Here's how the part is built. I have some questions about the finished solid (model axes, mm). A direction names the side the tool comes from. Coordinates: 2 decimals unless noted, no trailing zeros. Write each loop counter-clockwise with the first axis right and the second up, starting at its lowest first coordinate (ties: lowest second). Pieces come first, ordered by that corner, then holes. Notation, with made-up numbers: (32.25, 24) -> (50.25, 24) arc R21 cw to (50.25, 60) -> close; hole circle Ø1 at (40, -6). An arc over 180 degrees is marked (long way). Put each result on its own line as item: value.
```python
from build123d import *

# Parameters (mm, degrees)
BOX007_W                  = 50
BOX007_H                  = 58
BOX007_DEPTH              = 50
BOX006_W                  = 50
BOX006_H                  = 50
BOX006_DEPTH              = 50
CUT002008_PLACEMENT_ANGLE = 180


with BuildPart() as cube002:
    # Box007 → Box007 (new body)
    with BuildSketch(Plane(origin=(5, -3, -5), x_dir=(1, 0, 0), z_dir=(0, 0, 1))):
        with Locations((25, 29)):
            Rectangle(BOX007_W, BOX007_H)
    extrude(amount=BOX007_DEPTH)


with BuildPart() as cut002008:
    # Box006 → Box006 (new body)
    with BuildSketch(Plane.XY):
        with Locations((25, 25)):
            Rectangle(BOX006_W, BOX006_H)
    extrude(amount=BOX006_DEPTH)

    # Cut002008: cut Cube002
    add(cube002.part, mode=Mode.SUBTRACT)


with BuildPart() as cut002008_1:
    # Cut002008 placement: moved
    add(cut002008.part.moved(Location((66, 35, 56))).rotate(Axis((66, 35, 56), (0, 1, 0)), CUT002008_PLACEMENT_ANGLE))


solid = cut002008_1.part
```
Item 1: Imagine slicing it at C-C on z = 37. Write out the boundary of the cut face in (x, y).
Output:
outline: (61, 35) -> (66, 35) -> (66, 85) -> (61, 85) -> close
Item 2: Imagine slicing it at A-A on y = 41. Write out the boundary of the cut face in (x, z), then the cut area to 3 significant figures.
Output:
outline: (16, 6) -> (66, 6) -> (66, 56) -> (61, 56) -> (61, 11) -> (16, 11) -> close
area: 475 mm²
Item 3: Imagine slicing it at B-B on x = 35. Write out the boundary of the cut face in (y, z).
Output:
outline: (35, 6) -> (85, 6) -> (85, 11) -> (35, 11) -> close
Item 4: Please list where these lines run through material, in increasing order: line 1 along X through (y, z) = (50.5, 32.5); line 2 along Z through (x, y) = (19, 48). Write a range as from..to.
Output:
line 1: x = 61..66
line 2: z = 6..11
Item 5: For P1, Ø4, axis at x = 57.5, z = 49, coming from the -Y side; P2, Ø1, axis at y = 61, z = 32.5, coming from the -X side; P3, Ø12, axis at x = 26.5, y = 42, coming from the +Z side, each with a flat end and sliding along its axis, tell me the tip position at first contact or that it passes through.
Output:
P1: passes through
P2: stops at x = 61
P3: stops at z = 11
Item 6: Which directions (+Z, -Z, +X, -X, +Y, -Y) give clear straight access to the entire face, cutting with the end or side of a thin tool? Please do faces 1 (the flat face through (16, 60, 9)), 2 (the flat face through (61, 60, 34)).
Output:
face 1: +Z, -Z, -X, +Y, -Y
face 2: +Z, -X, +Y, -Y
